The listing builds one solid part. Answer for the finished solid, in the listing's coordinates (mm). A direction names the side the tool comes from. Give positions to 0.01 mm unless a question says otherwise; leave off trailing zeros. Order: outer loops, then holes, each group sorted by start corner. A loop starts at its lowest first (then second) coordinate and runs counter-clockwise, first axis right, second up. Notation, with made-up numbers: (28, 78.5) - (75, 78.5) arc R10 cw to (75, 90.5) - close; hole circle Ø7 at (38, 81.25). An arc over 180 degrees is marked (long way). Answer in a Markdown table with one row per item.
from build123d import *

# Parameters (mm, degrees)
F0_W       = 120
F0_H       = 13
F0_R       = 1.5
F1_DEPTH   = 3
F2_DEPTH   = 9
F3_DEPTH   = 12
F4_R       = 5
F5_SIZE2   = 1.5
F5_SIZE    = 2
F5_2_SIZE2 = 1.5
F5_2_SIZE  = 2
F5_3_SIZE2 = 1.5
F5_3_SIZE  = 2
F6_SIZE    = 1.5


with BuildPart() as f1:
    # F0 (on Top) → F1 (new body)
    with BuildSketch(Plane.XY):
        with Locations((40, 18.5)):
            Rectangle(F0_W, F0_H)
        with Locations((-10, 18.5)):
            Circle(F0_R, mode=Mode.SUBTRACT)
        with Locations((40, 18.5)):
            Circle(F0_R, mode=Mode.SUBTRACT)
        with Locations((90, 18.5)):
            Circle(F0_R, mode=Mode.SUBTRACT)
        Polygon((-20, 0), (0, 0), (80, 0), (100, 0), (100, 12), (-20, 12), align=None)
        with BuildLine():
            Line((0, -25), (0, 0))
            Line((0, 0), (-20, 0))
            Line((-20, 0), (-20, -34.5516387229))
            ThreePointArc((-20, -34.5516387229), (40, -45), (100, -34.5516387229))
            Line((100, -34.5516387229), (100, 0))
            Line((100, 0), (80, 0))
            Line((80, 0), (80, -25))
            ThreePointArc((80, -25), (40, -30), (0, -25))
        make_face()
    extrude(amount=F1_DEPTH)

    # F0 (on Top) → F2 (join)
    with BuildSketch(Plane.XY):
        with Locations((40, 18.5)):
            Rectangle(F0_W, F0_H)
        with Locations((-10, 18.5)):
            Circle(F0_R, mode=Mode.SUBTRACT)
        with Locations((40, 18.5)):
            Circle(F0_R, mode=Mode.SUBTRACT)
        with Locations((90, 18.5)):
            Circle(F0_R, mode=Mode.SUBTRACT)
    extrude(amount=-F2_DEPTH)

    # F0 (on Top) → F3 (join)
    with BuildSketch(Plane.XY):
        with BuildLine():
            Line((0, -25), (0, 0))
            Line((0, 0), (-20, 0))
            Line((-20, 0), (-20, -34.5516387229))
            ThreePointArc((-20, -34.5516387229), (40, -45), (100, -34.5516387229))
            Line((100, -34.5516387229), (100, 0))
            Line((100, 0), (80, 0))
            Line((80, 0), (80, -25))
            ThreePointArc((80, -25), (40, -30), (0, -25))
        make_face()
    extrude(amount=-F3_DEPTH)

    # F4
    f4_edges = [f1.edges().sort_by_distance(p)[0] for p in [
        (-20, -34.551639, -4.5),
        (100, -34.551639, -4.5),
        (0, 0, 1.5),
        (80, 0, 1.5),
        (80, -25, -4.5),
        (0, -25, -4.5),
        (100, 25, -3),
        (-20, 25, -3),
    ]]
    fillet(f4_edges, radius=F4_R)

    # F5
    f5_edges = [f1.edges().sort_by_distance(p)[0] for p in [
        (-11.5, 18.5, 3),
    ]]
    f5_side = f1.faces().sort_by_distance((-11.5, 18.5, -3))[0]
    chamfer(f5_edges, length=F5_SIZE, length2=F5_SIZE2, reference=f5_side)

    # F5#2
    f5_2_edges = [f1.edges().sort_by_distance(p)[0] for p in [
        (38.5, 18.5, 3),
    ]]
    f5_2_side = f1.faces().sort_by_distance((38.5, 18.5, -3))[0]
    chamfer(f5_2_edges, length=F5_2_SIZE, length2=F5_2_SIZE2, reference=f5_2_side)

    # F5#3
    f5_3_edges = [f1.edges().sort_by_distance(p)[0] for p in [
        (88.5, 18.5, 3),
    ]]
    f5_3_side = f1.faces().sort_by_distance((88.5, 18.5, -3))[0]
    chamfer(f5_3_edges, length=F5_3_SIZE, length2=F5_3_SIZE2, reference=f5_3_side)

    # F6
    f6_edges = [f1.edges().sort_by_distance(p)[0] for p in [
        (40, 0, 3),
        (-20, -5.498471, 3),
        (100, -15.498471, -12),
        (99.060235, -33.914902, -12),
        (90, 0, -12),
        (40, -45, -12),
        (80, -10.530938, -12),
        (-19.060235, -33.914902, -12),
        (78.90868, -24.179925, -12),
        (-20, -15.498471, -12),
        (40, -30, -12),
        (-10, 0, -12),
        (1.09132, -24.179925, -12),
        (0, -10.530938, -12),
        (40, 12, -9),
        (40, 25, -9),
    ]]
    chamfer(f6_edges, length=F6_SIZE)


solid = f1.part
Item 1: Find section B-B on y = -19. Write down the section's boundary in (x, z).
Answer block:
| item | result |
|---|---|
| outline | (-20, -10.5) - (-18.5, -12) - (-1.5, -12) - (0, -10.5) - (0, 1.5) - (-1.5, 3) - (-18.5, 3) - (-20, 1.5) - close; (80, -10.5) - (81.5, -12) - (98.5, -12) - (100, -10.5) - (100, 1.5) - (98.5, 3) - (81.5, 3) - (80, 1.5) - close |
Item 2: Find section C-C on x = 40. Write down the section's boundary in (y, z).
Answer block:
| item | result |
|---|---|
| outline | (-45, -10.5) - (-43.5, -12) - (-31.5, -12) - (-30, -10.5) - (-30, 1.5) - (-31.5, 3) - (-43.5, 3) - (-45, 1.5) - close; (0, 0) - (12, 0) - (12, -7.5) - (13.5, -9) - (17, -9) - (17, 1) - (15.5, 3) - (1.5, 3) - (0, 1.5) - close; (20, -9) - (23.5, -9) - (25, -7.5) - (25, 1.5) - (23.5, 3) - (21.5, 3) - (20, 1) - close |
Item 3: Which of the six approach directions +Z, -Z, +X, -X, +Y, -Y give full straight-line access (tool end or side, diameter ignored) to faces 1 (the face through (-10, 0, -5)), 2 (the face through (40.5, -30, -4.4)), 3 (the face through (39, 21, -9)), 4 (the face through (78.78, -1.135, 1.906)), 5 (the face through (0, -11, -4))?
Answer block:
| item | result |
|---|---|
| face 1 | -Z, +X, -X |
| face 2 | +Z, -Z |
| face 3 | -Z, +X, -X, +Y |
| face 4 | +Z |
| face 5 | -Z |
Item 4: Each of these flat-tipped pins is pushed along its axis until it touches: P1, Ø2.5, axis at x = 40, y = 18.5, coming from the +Z side; P2, Ø5, axis at x = 90, y = 18.5, coming from the +Z side; P3, Ø1.5, axis at x = 0.5, y = -24, coming from the -Z side; P4, Ø5, axis at x = 50.5, y = -29.5, coming from the +Z side. Where does it stop, or does it pass through?
Answer block:
| item | result |
|---|---|
| P1 | through |
| P2 | z = 2.33 |
| P3 | z = -11.62 |
| P4 | z = 3 |
Item 5: Find section D-D on y = 18.5. Write down the section's boundary in (x, z).
Answer block:
| item | result |
|---|---|
| outline | (-20, -7.5) - (-18.5, -9) - (-11.5, -9) - (-11.5, 1) - (-13, 3) - (-18.5, 3) - (-20, 1.5) - close; (-8.5, -9) - (38.5, -9) - (38.5, 1) - (37, 3) - (-7, 3) - (-8.5, 1) - close; (41.5, -9) - (88.5, -9) - (88.5, 1) - (87, 3) - (43, 3) - (41.5, 1) - close; (91.5, -9) - (98.5, -9) - (100, -7.5) - (100, 1.5) - (98.5, 3) - (93, 3) - (91.5, 1) - close |
Item 6: Determine the mould class of faces 6 (the face through (90, 0, -5)), 7 (the face through (38.89, 19.51, -4.07)), 8 (the face through (-20, -11, -4)) for opening direction X: pulls with the +X half, pulls with the -X half, needs draft (parallel to the pull), parting line crosses it, or undercut.
Answer block:
| item | result |
|---|---|
| face 6 | needs draft |
| face 7 | undercut |
| face 8 | pulls with the -X half |
Item 7: Find section A-A on z = -2.25. Write down the section's boundary in (x, y), then the cut area to 3 significant figures.
Answer block:
| item | result |
|---|---|
| outline | (-20, -31) arc R5 ccw to (-16.59, -35.74) arc R177.5 ccw to (96.59, -35.74) arc R5 ccw to (100, -31) - (100, 0) - (80, 0) - (80, -21.06) arc R5 cw to (76.11, -25.94) arc R162.5 cw to (3.89, -25.94) arc R5 cw to (0, -21.06) - (0, 0) - (-20, 0) - close; (-20, 12) - (100, 12) - (100, 20) arc R5 ccw to (95, 25) - (-15, 25) arc R5 ccw to (-20, 20) - close; hole circle Ø3 at (-10, 18.5); hole circle Ø3 at (40, 18.5); hole circle Ø3 at (90, 18.5) |
| area | 4,250 mm² |
Item 8: Consider line 1 (Y direction, x = 40, z = -5.75); line 2 (X direction, y = -4, z = -8.25); line 3 (Y direction, x = 89, z = -8). Determine where each line is inside the solid, lowest interval first.
Answer block:
| item | result |
|---|---|
| line 1 | -45 to -30, 12 to 17, 20 to 25 |
| line 2 | -20 to 0, 80 to 100 |
| line 3 | -38.1 to 0, 12.5 to 17.38, 19.62 to 24.5 |
